Check sheet for the modelled part. Datum: model origin and axes. Units: mm. Round coordinates to 2 decimals unless told otherwise and drop trailing zeros. Write each loop counter-clockwise with the first axis right and the second up, starting at its lowest first coordinate (ties: lowest second). Pieces come first, ordered by that corner, then holes. Notation, with made-up numbers: (-33.5, 56) -> (14.5, 56) arc R12 ccw to (14.5, 79) -> close; hole circle Ø10 at (-16.75, 23). An arc over 180 degrees is marked (long way). Write item = value, one per line.
from build123d import *

# Parameters (mm, degrees)
SKETCH1_W           = 120
SKETCH1_H           = 100
BOSS_EXTRUDE1_DEPTH = 10
SKETCH2_W           = 98.5
SKETCH2_H           = 40
CUT_EXTRUDE1_DEPTH  = 10
SKETCH3_W           = 120
SKETCH3_H           = 100
SKETCH3_W_2         = 111.2
SKETCH3_H_2         = 91.2
CUT_EXTRUDE3_DEPTH  = 7
SKETCH4_W           = 18
SKETCH4_H           = 25
CUT_EXTRUDE4_DEPTH  = 8
SKETCH5_W           = 3
SKETCH5_H           = 25
CUT_EXTRUDE6_DEPTH  = 1
SKETCH6_R           = 4
CUT_EXTRUDE12_DEPTH = 81.067810822
SKETCH7_W           = 45.061320755
SKETCH7_H           = 5
CUT_EXTRUDE13_DEPTH = 2


with BuildPart() as part:
    # Sketch1 → Boss-Extrude1 (new body)
    with BuildSketch(Plane(origin=(0, 0, 0), x_dir=(1, 0, 0), z_dir=(0, 1, 0))):
        with Locations((0.311320755, 2.051886792)):
            Rectangle(SKETCH1_W, SKETCH1_H)
    extrude(amount=BOSS_EXTRUDE1_DEPTH)

    # Sketch2 → Cut-Extrude1 (cut)
    with BuildSketch(Plane(origin=(0, 10, 0), x_dir=(1, 0, 0), z_dir=(0, 1, 0))):
        with Locations((0.811320755, 17.051886792)):
            Rectangle(SKETCH2_W, SKETCH2_H)
    extrude(amount=-CUT_EXTRUDE1_DEPTH, mode=Mode.SUBTRACT)

    # Sketch3 → Cut-Extrude3 (cut)
    with BuildSketch(Plane.XZ):
        with Locations((0.311320755, -2.051886792)):
            Rectangle(SKETCH3_W, SKETCH3_H)
        with Locations((0.311320755, -2.051886792)):
            Rectangle(SKETCH3_W_2, SKETCH3_H_2, mode=Mode.SUBTRACT)
    extrude(amount=-CUT_EXTRUDE3_DEPTH, mode=Mode.SUBTRACT)

    # Sketch4 → Cut-Extrude4 (cut)
    with BuildSketch(Plane.XZ):
        with Locations((-39.17934754, 27.448113208)):
            Rectangle(SKETCH4_W, SKETCH4_H)
        with Locations((-19.133803456, 27.448113208)):
            Rectangle(SKETCH4_W, SKETCH4_H)
        with Locations((0.911740628, 27.448113208)):
            Rectangle(SKETCH4_W, SKETCH4_H)
        with Locations((20.957284712, 27.448113208)):
            Rectangle(SKETCH4_W, SKETCH4_H)
        with Locations((41.002828796, 27.448113208)):
            Rectangle(SKETCH4_W, SKETCH4_H)
    extrude(amount=-CUT_EXTRUDE4_DEPTH, mode=Mode.SUBTRACT)

    # Sketch5 → Cut-Extrude6 (cut)
    with BuildSketch(Plane.XZ.offset(-8)):
        with Locations((33.502828796, 27.448113208)):
            Rectangle(SKETCH5_W, SKETCH5_H)
        with Locations((13.457284712, 27.448113208)):
            Rectangle(SKETCH5_W, SKETCH5_H)
        with Locations((-6.588259372, 27.448113208)):
            Rectangle(SKETCH5_W, SKETCH5_H)
        with Locations((-26.633803456, 27.448113208)):
            Rectangle(SKETCH5_W, SKETCH5_H)
        with Locations((-46.67934754, 27.448113208)):
            Rectangle(SKETCH5_W, SKETCH5_H)
    extrude(amount=-CUT_EXTRUDE6_DEPTH, mode=Mode.SUBTRACT)

    # Sketch6 → Cut-Extrude12 (cut, through all)
    with BuildSketch(Plane.XZ.offset(-8)):
        with Locations(Location((41.502828796, 24.198113208, 0), (0, 0, 270))):
            Circle(SKETCH6_R)
        with Locations(Location((21.457284712, 24.198113208, 0), (0, 0, 270))):
            Circle(SKETCH6_R)
        with Locations(Location((1.411740628, 24.198113208, 0), (0, 0, 270))):
            Circle(SKETCH6_R)
        with Locations(Location((-18.633803456, 24.198113208, 0), (0, 0, 270))):
            Circle(SKETCH6_R)
        with Locations(Location((-38.67934754, 24.198113208, 0), (0, 0, 270))):
            Circle(SKETCH6_R)
    extrude(amount=-CUT_EXTRUDE12_DEPTH, mode=Mode.SUBTRACT)

    # Sketch7 → Cut-Extrude13 (cut)
    with BuildSketch(Plane.XZ):
        with Locations((22.530660378, -39.551886792)):
            Rectangle(SKETCH7_W, SKETCH7_H)
    extrude(amount=-CUT_EXTRUDE13_DEPTH, mode=Mode.SUBTRACT)


solid = part.part
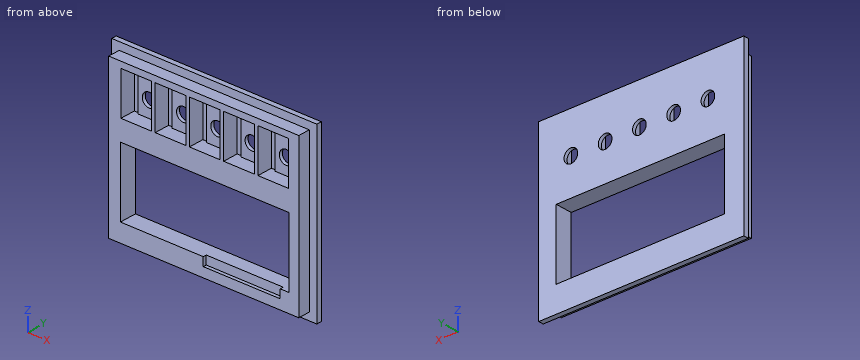
(1) Sectioned sample at B-B on y = 4.5. Enter the section's corners in (x, z), then the cut area to 3 significant figures.
Worked answers:
outline = (-55.29, -47.65) -> (55.91, -47.65) -> (55.91, 43.55) -> (-55.29, 43.55) -> close; hole (-48.44, -37.05) -> (50.06, -37.05) -> (50.06, 2.95) -> (-48.44, 2.95) -> close; hole (-48.18, 14.95) -> (-30.18, 14.95) -> (-30.18, 39.95) -> (-48.18, 39.95) -> close; hole (-28.13, 14.95) -> (-10.13, 14.95) -> (-10.13, 39.95) -> (-28.13, 39.95) -> close; hole (-8.09, 14.95) -> (9.91, 14.95) -> (9.91, 39.95) -> (-8.09, 39.95) -> close; hole (11.96, 14.95) -> (29.96, 14.95) -> (29.96, 39.95) -> (11.96, 39.95) -> close; hole (32, 14.95) -> (50, 14.95) -> (50, 39.95) -> (32, 39.95) -> close
area = 3,950 mm²
(2) Sectioned sample at D-D on x = 3. Enter the section's corners in (y, z), then the cut area to 3 significant figures.
Worked answers:
outline = (0, -47.65) -> (7, -47.65) -> (7, -52.05) -> (10, -52.05) -> (10, -37.05) -> (2, -37.05) -> (2, -42.05) -> (0, -42.05) -> close; (0, 2.95) -> (10, 2.95) -> (10, 20.53) -> (8, 20.53) -> (8, 14.95) -> (0, 14.95) -> close; (0, 39.95) -> (8, 39.95) -> (8, 27.87) -> (10, 27.87) -> (10, 47.95) -> (7, 47.95) -> (7, 43.55) -> (0, 43.55) -> close
area = 314 mm²
(3) Sectioned sample at C-C on x = 43.5. Enter the section's corners in (y, z), then the cut area to 3 significant figures.
Worked answers:
outline = (0, -47.65) -> (7, -47.65) -> (7, -52.05) -> (10, -52.05) -> (10, -37.05) -> (2, -37.05) -> (2, -42.05) -> (0, -42.05) -> close; (0, 2.95) -> (10, 2.95) -> (10, 20.73) -> (8, 20.73) -> (8, 14.95) -> (0, 14.95) -> close; (0, 39.95) -> (8, 39.95) -> (8, 27.66) -> (10, 27.66) -> (10, 47.95) -> (7, 47.95) -> (7, 43.55) -> (0, 43.55) -> close
area = 315 mm²
(4) Sectioned sample at A-A on x = 28.5. Enter the section's corners in (y, z).
Worked answers:
outline = (0, -47.65) -> (7, -47.65) -> (7, -52.05) -> (10, -52.05) -> (10, -37.05) -> (2, -37.05) -> (2, -42.05) -> (0, -42.05) -> close; (0, 2.95) -> (10, 2.95) -> (10, 47.95) -> (7, 47.95) -> (7, 43.55) -> (0, 43.55) -> (0, 39.95) -> (8, 39.95) -> (8, 14.95) -> (0, 14.95) -> close
(5) Go/stop test with flat-tipped pins: P1, Ø12, axis at x = -37, z = 21.5, coming from the -Y side; P2, Ø4.5, axis at x = -34.5, y = 3, coming from the -Z side; P3, Ø1.6, axis at y = 1.5, z = -39.5, coming from the +X side. Record where each tip stops, or that it passes through.
Worked answers:
P1 = 8
P2 = -47.65
P3 = 55.91
(6) Material ranges on L1, parallel to X at y = 5.5, z = 25; L2, parallel to Z at x = 2.5, y = 7.5; L3, parallel to Z at x = 21.5, y = 4.25, recorded low to high. Write a range as [from, to].
Worked answers:
L1 = [-55.29, -48.18], [-30.18, -28.13], [-10.13, -8.09], [9.91, 11.96], [29.96, 32], [50, 55.91]
L2 = [-52.05, -37.05], [2.95, 14.95], [39.95, 47.95]
L3 = [-47.65, -37.05], [2.95, 14.95], [39.95, 43.55]
